The listing builds one solid part. Answer for the finished solid, in the listing's coordinates (mm). A direction names the side the tool comes from. Give positions to 0.01 mm unless a question says otherwise; leave off trailing zeros. Loops run counter-clockwise (first coordinate to the right, second up) from the corner with the lowest first, then second, coordinate; pieces in that order, holes last. Notation, with made-up numbers: M 66,14 L 124,14 A10 cw 124,27 Z; hole C -22.5,4.25 d1. An arc over 180 degrees is marked long. Return JSON: item names as keys, results as strings.
from build123d import *

# Parameters (mm, degrees)
F0_R     = 6.25
F1_DEPTH = 1.8
F3_DEPTH = 2
F4_SIZE  = 0.2


with BuildPart() as f1:
    # F0 (on Top) → F1 (new body)
    with BuildSketch(Plane.XY):
        Circle(F0_R)
    extrude(amount=F1_DEPTH)

    # F2 (on face) → F3 (join)
    with BuildSketch(Plane.XY.offset(1.8)):
        with BuildLine():
            Line((2.472136, -3.402603), (0, 4.205849))
            Line((0, 4.205849), (-2.472136, -3.402603))
            ThreePointArc((-2.472136, -3.402603), (0, -3.794151), (2.472136, -3.402603))
        make_face()
    extrude(amount=F3_DEPTH)

    # F4
    f4_edges = [f1.edges().sort_by_distance(p)[0] for p in [
        (-6.25, 0, 0),
    ]]
    chamfer(f4_edges, length=F4_SIZE)


solid = f1.part
(1) The part is cut by section A-A (y = 0). Determine the outline of the cut face in (x, z), and give its area (3 significant figures).
Values follow:
{"outline": "M -6.25,0.2 L -6.05,0 L 6.05,0 L 6.25,0.2 L 6.25,1.8 L 1.37,1.8 L 1.37,3.8 L -1.37,3.8 L -1.37,1.8 L -6.25,1.8 Z", "area": "27.9 mm²"}
(2) Given pin 1 (5 mm diameter, centred on x = 4, y = 4, fed in from +Z), flat-ended and moving along its own axis, determine where the tip first touches the part or whether it passes through.
Values follow:
{"pin 1": "z = 1.8"}
(3) Straight lines are drawn through the part: line 1 along Z through (x, y) = (-3, -0.75); line 2 along X through (y, z) = (-3, 2.9); line 3 along Y through (x, z) = (-0.5, 0.75). For each, find the intervals that lie inside material, in ascending order.
Values follow:
{"line 1": "0 to 1.8", "line 2": "-2.34 to 2.34", "line 3": "-6.23 to 6.23"}
(4) The part is cut by section B-B (z = 1.3). Determine the outline of the cut face in (x, y), and give its area (3 significant figures).
Values follow:
{"outline": "C 0,0 d12.5", "area": "123 mm²"}
(5) Determine the mould class of faces 1 (the flat face through (0, 0, 0)), 2 (the cylindrical face through (5.96, 1.88, 0.99)), 3 (the flat face through (1.253, 0.348, 2.786)) for opening direction X: released by +X, released by -X, zero draft, split by the parting line, or undercut.
Values follow:
{"face 1": "zero draft", "face 2": "split by the parting line", "face 3": "released by +X"}
(6) A tool of negligible diameter and unlimited length cuts with its end or side. For faces 4 (the flat face through (0, -1, 3.8)), 5 (the cylindrical face through (-0.035, -3.794, 2.786)), 6 (the flat face through (-1.22, 0.45, 2.79)), from which of +Z, -Z, +X, -X, +Y, -Y can it reach the whole face along a straight path? Write none if from no direction.
Values follow:
{"face 4": "+Z, +X, -X, +Y, -Y", "face 5": "+Z, -Y", "face 6": "+Z, -X, +Y"}
(7) The part is cut by section C-C (z = 2.2). Determine the outline of the cut face in (x, y), and give its area (3 significant figures).
Values follow:
{"outline": "M -2.47,-3.4 A8 ccw 2.47,-3.4 L 0,4.21 Z", "area": "20.1 mm²"}
